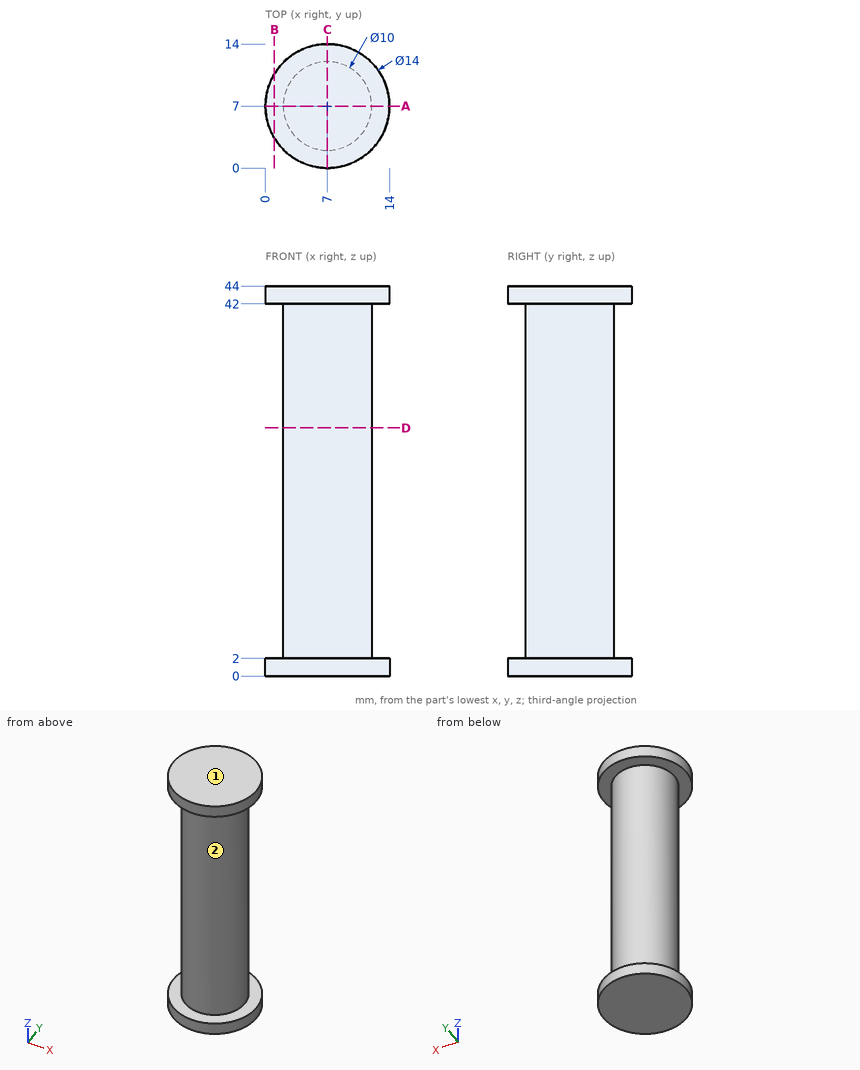
The figure shows three views and two pictorial views of one solid part (mm, origin at its lowest corner). Answer the questions. A direction names the side the tool comes from. Round coordinates to 2 decimals unless told otherwise and drop trailing zeros. Loops run counter-clockwise (first coordinate to the right, second up) from the corner with the lowest first, then second, coordinate; pieces in that order, holes last. Notation, with made-up numbers: (61.25, -8.75) - (73.25, -8.75) arc R22 ccw to (73.25, 8.25) - close; hole circle Ø8 at (-4, 15). An arc over 180 degrees is marked (long way). One line per question, with ' | ' between items. Start each with the question number.
Q1. Section A-A on y = 7 is taken. Give the vertices of the cut face in (x, z), plus the area to 3 significant figures.
Q2. Section D-D on z = 28 is taken. Give the vertices of the cut face in (x, y).
Q3. Section B-B on x = 1 is taken. Give the vertices of the cut face in (y, z).
Q4. For the marked faces 1 and 2, determine the directions among +Z, -Z, +X, -X, +Y, -Y from which every point of the face is accessible in a straight line to the end or side of a thin tool.
Q5. Flat-ended cylindrical pins translate along their axes: pin 1 (4 mm diameter, centred on y = 8, z = 23.5, fed in from +X); pin 2 (2 mm diameter, centred on x = 7, z = 5.5, fed in from +Y); pin 3 (6 mm diameter, centred on x = 10, z = 9, fed in from -Y). Find the tip coordinate at first contact, or state that the pin passes through.
Q6. Find the intervals of material crossed by L1, parallel to Z at x = 13.25, y = 4.75; L2, parallel to Y at x = 7, z = 38.5; L3, parallel to Y at x = 4.5, z = 26.5, in increasing order.
Established:
1) outline: (0, 0) - (14, 0) - (14, 2) - (12, 2) - (12, 42) - (14, 42) - (14, 44) - (0, 44) - (0, 42) - (2, 42) - (2, 2) - (0, 2) - close | area: 456 mm²
2) outline: circle Ø10 at (7, 7)
3) outline: (3.39, 0) - (10.61, 0) - (10.61, 2) - (3.39, 2) - close; (3.39, 42) - (10.61, 42) - (10.61, 44) - (3.39, 44) - close
4) face 1: +Z, +X, -X, +Y, -Y | face 2: none
5) pin 1: x = 12 | pin 2: y = 12 | pin 3: y = 2
6) L1: 0 to 2, 42 to 44 | L2: 2 to 12 | L3: 2.67 to 11.33
